from build123d import *

# Parameters (mm, degrees)
ESQUISSE1_R             = 8
BOSS_EXTRU_1_DEPTH      = 4.9
BOSS_EXTRU_2_START      = 1.5
BOSS_EXTRU_2_DEPTH      = 1.5
BOSS_EXTRU_3_DEPTH      = 51.5
ENL_V_MAT_EXTRU_1_DEPTH = 25


with BuildPart() as part:
    # Esquisse1 → Boss.-Extru.1 (new body)
    with BuildSketch(Plane.XY):
        with Locations((-10.25, -10)):
            Circle(ESQUISSE1_R)
        with BuildLine():
            Line((-5.751675839, -9.877200395), (-6.833750507, -9.782531128))
            Line((-6.833750507, -9.782531128), (-6.949445107, -9.126394451))
            Line((-6.949445107, -9.126394451), (-5.953521963, -8.661987862))
            ThreePointArc((-5.953521963, -8.661987862), (-6.006634107, -8.502052772), (-6.065697468, -8.344218516))
            Line((-6.065697468, -8.344218516), (-7.138261768, -8.631611254))
            Line((-7.138261768, -8.631611254), (-7.47139109, -8.054614344))
            Line((-7.47139109, -8.054614344), (-6.678798898, -7.262022153))
            ThreePointArc((-6.678798898, -7.262022153), (-6.782621037, -7.131675902), (-6.891198054, -7.005263035))
            Line((-6.891198054, -7.005263035), (-7.818046533, -7.654249327))
            Line((-7.818046533, -7.654249327), (-8.328430264, -7.225986526))
            Line((-8.328430264, -7.225986526), (-7.847635402, -6.194918616))
            ThreePointArc((-7.847635402, -6.194918616), (-7.988951343, -6.109285545), (-8.133315872, -6.028898352))
            Line((-8.133315872, -6.028898352), (-8.791112727, -6.968329619))
            Line((-8.791112727, -6.968329619), (-9.417191057, -6.740455742))
            Line((-9.417191057, -6.740455742), (-9.317216173, -5.597737589))
            ThreePointArc((-9.317216173, -5.597737589), (-9.478728542, -5.566588183), (-9.641271425, -5.541362369))
            Line((-9.641271425, -5.541362369), (-9.940094206, -6.656584169))
            Line((-9.940094206, -6.656584169), (-10.606352849, -6.656584169))
            Line((-10.606352849, -6.656584169), (-10.903477232, -5.547700874))
            ThreePointArc((-10.903477232, -5.547700874), (-11.065761738, -5.574558464), (-11.226956242, -5.607329229))
            Line((-11.226956242, -5.607329229), (-11.126406846, -6.756614081))
            Line((-11.126406846, -6.756614081), (-11.752485176, -6.984487958))
            Line((-11.752485176, -6.984487958), (-12.406540122, -6.050400691))
            ThreePointArc((-12.406540122, -6.050400691), (-12.550096477, -6.132241451), (-12.690551241, -6.219297732))
            Line((-12.690551241, -6.219297732), (-12.206963835, -7.256354271))
            Line((-12.206963835, -7.256354271), (-12.717347566, -7.684617071))
            Line((-12.717347566, -7.684617071), (-13.638885709, -7.039349117))
            ThreePointArc((-13.638885709, -7.039349117), (-13.74618945, -7.166864047), (-13.848697947, -7.298264801))
            Line((-13.848697947, -7.298264801), (-13.051434053, -8.095528695))
            Line((-13.051434053, -8.095528695), (-13.384563375, -8.672525605))
            Line((-13.384563375, -8.672525605), (-14.450903238, -8.3868007))
            ThreePointArc((-14.450903238, -8.3868007), (-14.508366703, -8.545244687), (-14.559856563, -8.705729393))
            Line((-14.559856563, -8.705729393), (-13.557961929, -9.172920534))
            Line((-13.557961929, -9.172920534), (-13.673656528, -9.829057211))
            Line((-13.673656528, -9.829057211), (-14.74934404, -9.923167674))
            ThreePointArc((-14.74934404, -9.923167674), (-14.749021481, -10.093838761), (-14.74222728, -10.264374865))
            Line((-14.74222728, -10.264374865), (-13.665452724, -10.358580432))
            Line((-13.665452724, -10.358580432), (-13.549758125, -11.014717109))
            Line((-13.549758125, -11.014717109), (-14.506309194, -11.460764198))
            ThreePointArc((-14.506309194, -11.460764198), (-14.447094307, -11.623083293), (-14.381691786, -11.78300953))
            Line((-14.381691786, -11.78300953), (-13.360941463, -11.509500306))
            Line((-13.360941463, -11.509500306), (-13.027812142, -12.086497216))
            Line((-13.027812142, -12.086497216), (-13.758807936, -12.817493011))
            ThreePointArc((-13.758807936, -12.817493011), (-13.646852578, -12.951506829), (-13.529782028, -13.081076086))
            Line((-13.529782028, -13.081076086), (-12.681156698, -12.486862233))
            Line((-12.681156698, -12.486862233), (-12.170772967, -12.915125033))
            Line((-12.170772967, -12.915125033), (-12.600738895, -13.837189942))
            ThreePointArc((-12.600738895, -13.837189942), (-12.448909121, -13.926168447), (-12.293716433, -14.009142444))
            Line((-12.293716433, -14.009142444), (-11.708090504, -13.172781941))
            Line((-11.708090504, -13.172781941), (-11.082012174, -13.400655818))
            Line((-11.082012174, -13.400655818), (-11.169878896, -14.404977051))
            ThreePointArc((-11.169878896, -14.404977051), (-10.996236031, -14.437694422), (-10.821442589, -14.463569577))
            Line((-10.821442589, -14.463569577), (-10.559109026, -13.48452739))
            Line((-10.559109026, -13.48452739), (-9.892850383, -13.48452739))
            Line((-9.892850383, -13.48452739), (-9.632173683, -14.457386077))
            ThreePointArc((-9.632173683, -14.457386077), (-9.45766281, -14.42969545), (-9.284373537, -14.395175256))
            Line((-9.284373537, -14.395175256), (-9.372796385, -13.384497479))
            Line((-9.372796385, -13.384497479), (-8.746718055, -13.156623602))
            Line((-8.746718055, -13.156623602), (-8.164782025, -13.987714383))
            ThreePointArc((-8.164782025, -13.987714383), (-8.010469052, -13.903139907), (-7.859580663, -13.812596936))
            Line((-7.859580663, -13.812596936), (-8.292239396, -12.884757289))
            Line((-8.292239396, -12.884757289), (-7.781855665, -12.456494489))
            Line((-7.781855665, -12.456494489), (-6.938532496, -13.046995729))
            ThreePointArc((-6.938532496, -13.046995729), (-6.822819391, -12.916236114), (-6.712266113, -12.78108593))
            Line((-6.712266113, -12.78108593), (-7.447769178, -12.045582865))
            Line((-7.447769178, -12.045582865), (-7.114639857, -11.468585954))
            Line((-7.114639857, -11.468585954), (-6.100183444, -11.740408731))
            ThreePointArc((-6.100183444, -11.740408731), (-6.036436962, -11.579837499), (-5.978900904, -11.416937723))
            Line((-5.978900904, -11.416937723), (-6.941241303, -10.968191026))
            Line((-6.941241303, -10.968191026), (-6.825546704, -10.312054348))
            Line((-6.825546704, -10.312054348), (-5.755303948, -10.21842024))
            ThreePointArc((-5.755303948, -10.21842024), (-5.750254354, -10.04784472), (-5.751675839, -9.877200395))
        make_face(mode=Mode.SUBTRACT)
    extrude(amount=-BOSS_EXTRU_1_DEPTH)

    # Esquisse2 → Boss.-Extru.2 (add)
    with BuildSketch(Plane.XY.offset(BOSS_EXTRU_2_START)):
        with BuildLine():
            ThreePointArc((-3.303360096, -6.032104583), (-13.772784459, -2.817382813), (-17.640109889, -13.06370296))
            Line((-17.640109889, -13.06370296), (-17.639263276, -13.065744321))
            ThreePointArc((-17.639263276, -13.065744321), (43.56377057, -128.719994734), (125.190682292, -230.988094713))
            Line((125.190682292, -230.988094713), (-3.303360096, -6.032104583))
        make_face()
    extrude(amount=-BOSS_EXTRU_2_DEPTH)

    # Esquisse3 → Boss.-Extru.3 (add)
    with BuildSketch(Plane(origin=(0, 0, 0), x_dir=(-1, 0, 0), z_dir=(0, 0, -1))):
        with BuildLine():
            Line((-16.135278154, -40.063550967), (-125.190682292, -230.988094713))
            ThreePointArc((-125.190682292, -230.988094713), (-54.599179759, -145.051819269), (1.516379631, -49.034905857))
            ThreePointArc((1.516379631, -49.034905857), (-7.873342973, -45.658721787), (-16.135278154, -40.063550967))
        make_face()
    extrude(amount=BOSS_EXTRU_3_DEPTH)

    # Esquisse4 → Enlèv. mat.-Extru.1 (cut)
    with BuildSketch(Plane(origin=(-5.088632244, -2.906608208, 0), x_dir=(0, 0, -1), z_dir=(0.8683299880241373, 0.4959869271442563, 0))):
        with BuildLine():
            Line((-1.5, -3.599433877), (-1.5, -262.666831333))
            Line((-1.5, -262.666831333), (25, -262.666831333))
            ThreePointArc((25, -262.666831333), (5.142239669, -133.809040305), (-1.5, -3.599433877))
        make_face()
        with BuildLine():
            ThreePointArc((50.899666007, -42.791269762), (42.714152109, -153.29025104), (25, -262.666831333))
            Line((25, -262.666831333), (51.5, -262.666831333))
            Line((51.5, -262.666831333), (51.5, -42.791269762))
            Line((51.5, -42.791269762), (50.899666007, -42.791269762))
        make_face()
    extrude(amount=-ENL_V_MAT_EXTRU_1_DEPTH, mode=Mode.SUBTRACT)


solid = part.part
The model under review builds one solid part; all positions refer to its coordinate system, in mm. A direction names the side the tool comes from. Round coordinates to 2 decimals unless told otherwise and drop trailing zeros. One line per question, with ' | ' between items. Start each with the question number.
Item 1: Wall thickness on line 1 along Y through (x, z) = (2, -29); line 2 along X through (y, z) = (-106, -22.5); line 3 along Y through (x, z) = (53, -28): over which ranges is each line inside the solid? List them lowest first. Write a range as [from, to].
Item 2: For pin 1 (10 mm diameter, centred on x = -12, y = -9, fed in from -Z); pin 2 (1.5 mm diameter, centred on x = 12, z = -5.5, fed in from +Y); pin 3 (2 mm diameter, centred on y = -142, z = -25, fed in from -X); pin 4 (12 mm diameter, centred on x = 69, y = -118.5, fed in from -Z), all flat-tipped, find the tip position at first contact; note any pin that passes through.
Item 3: Draft analysis for pull direction Y (two halves, no side actions). For faces 3 (the face through (-1, -32, 0)), 4 (the face through (50.65, -117.63, -45.51)), 5 (the face through (-10, -10, 0)), state which applies: +Y half, -Y half, draft (parallel to the pull), parting line (faces both ways), or undercut.
Item 4: Machinability: for faces 1 (the face through (-13, -7, 1.5)), 2 (the face through (7.75, -45.72, -25.39)), which of the approach directions +Z, -Z, +X, -X, +Y, -Y give a long, thin tool a straight path to every point of the face, cutting with its end or side? Answer none if there is none.
Return value:
1) line 1: y = [-56.22, -48.08] | line 2: x = [29.29, 53.8] | line 3: y = [-142.75, -104.6]
2) pin 1: stops at z = -4.9 | pin 2: stops at y = -42.73 | pin 3: stops at x = 51.8 | pin 4: passes through
3) face 3: draft | face 4: -Y half | face 5: undercut
4) face 1: +Z, +X, -X, +Y, -Y | face 2: -Z, -X, +Y
